```python
from build123d import *

# Parameters (mm, degrees)
SKETCH1_W           = 20
SKETCH1_H           = 13
BOSS_EXTRUDE1_DEPTH = 3
SKETCH2_W           = 20
SKETCH2_H           = 3
BOSS_EXTRUDE2_DEPTH = 13
BOSS_EXTRUDE3_DEPTH = 3
CUT_EXTRUDE1_DEPTH  = 40.66221139


with BuildPart() as part:
    # Sketch1 → Boss-Extrude1 (new body)
    with BuildSketch(Plane.XY):
        with Locations((24.886831503, -27.055)):
            Rectangle(SKETCH1_W, SKETCH1_H)
    extrude(amount=BOSS_EXTRUDE1_DEPTH)

    # Sketch2 → Boss-Extrude2 (add)
    with BuildSketch(Plane.XY.offset(3)):
        with Locations((24.886831503, -22.055)):
            Rectangle(SKETCH2_W, SKETCH2_H)
    extrude(amount=BOSS_EXTRUDE2_DEPTH)

    # Sketch3 → Boss-Extrude3 (add)
    with BuildSketch(Plane(origin=(34.886831503, 0, 0), x_dir=(0, 0, -1), z_dir=(1, 0, 0))):
        Polygon((-7.239132511, -23.555), (-3, -27.79413251), (-3, -23.554999999), align=None)
    boss_extrude3 = extrude(amount=-BOSS_EXTRUDE3_DEPTH)

    # Sketch4 → Cut-Extrude1 (cut, through all)
    with BuildSketch(Plane.XZ.offset(23.555)):
        with BuildLine():
            Line((28.386831503, 4.812110779), (28.386831503, 13.441160462))
            ThreePointArc((28.386831503, 13.441160462), (29.886831503, 14.941160462), (31.386831503, 13.441160462))
            Line((31.386831503, 13.441160462), (31.386831503, 4.812110779))
            ThreePointArc((31.386831503, 4.812110779), (29.886831503, 3.312110779), (28.386831503, 4.812110779))
        make_face()
    cut_extrude1 = extrude(amount=-CUT_EXTRUDE1_DEPTH, mode=Mode.SUBTRACT)

    # Mirror1: Boss-Extrude3, Cut-Extrude1 across plane
    add(boss_extrude3.mirror(Plane.ZY.offset(-24.886831503)))
    add(cut_extrude1.mirror(Plane.ZY.offset(-24.886831503)), mode=Mode.SUBTRACT)


solid = part.part
```
Check sheet for the modelled part. Datum: model origin and axes. Units: mm. A direction names the side the tool comes from. Round coordinates to 2 decimals unless told otherwise and drop trailing zeros. Order: outer loops, then holes, each group sorted by start corner. A loop starts at its lowest first (then second) coordinate and runs counter-clockwise, first axis right, second up.
1) Section check A-A (y = -23.25). Record the boundary of the cut face in (x, z).
2) Section check C-C (x = 20.5). Record the boundary of the cut face in (y, z) (3 decimals).
3) Go/stop test with a flat-tipped pin: pin 1 Ø4 at (x, z) = (29.5, 9.5) entering from -Y (3 decimals). Record where the tip stops, or that it passes through.
4) Tool access check on faces 4 (the flat face through (28.387, -22, 9)), 5 (the flat face through (25, -23.555, 9)), 6 (the flat face through (25, -20.555, 8)). Record the directions out of +Z, -Z, +X, -X, +Y, -Y that give a thin tool (end or side, any length) a straight path to the whole face; none if there is none.
5) Scan lines: line 1 (X direction, y = -23, z = 4.75); line 2 (X direction, y = -24.5, z = 4); line 3 (Z direction, x = 22.5, y = -29.5). Record each from-to range of solid material in increasing order.
6) Section check B-B (z = 12). Record the boundary of the cut face in (x, y) (3 decimals).
7) Section check D-D (x = 33.25). Record the boundary of the cut face in (y, z) (3 decimals).
8) Mould release check, pull along X, two halves, no side actions. Record for faces 1 (the cylindrical face through (29.85, -22.08, 14.94)), 2 (the flat face through (16.366, -25.645, 5.149)), 3 (the flat face through (34.887, -24, 5)): +X half, -X half, draft (parallel to the pull), parting line (faces both ways), or undercut.
Result:
1. outline: (14.89, 0) - (34.89, 0) - (34.89, 16) - (14.89, 16) - close; hole (18.39, 4.81) arc R1.5 ccw to (21.39, 4.81) - (21.39, 13.44) arc R1.5 ccw to (18.39, 13.44) - close; hole (28.39, 4.81) arc R1.5 ccw to (31.39, 4.81) - (31.39, 13.44) arc R1.5 ccw to (28.39, 13.44) - close
2. outline: (-33.555, 0) - (-20.555, 0) - (-20.555, 3.443) - (-23.555, 3.443) - (-23.555, 3) - (-33.555, 3) - close; (-23.555, 14.81) - (-20.555, 14.81) - (-20.555, 16) - (-23.555, 16) - close
3. pin 1: stops at y = -23.555
4. face 4: +Y, -Y
4. face 5: +Z, -Y
4. face 6: +Z, -Z, +X, -X, +Y
5. line 1: x = 14.89 to 18.39, 21.39 to 28.39, 31.39 to 34.89
5. line 2: x = 14.89 to 17.89, 31.89 to 34.89
5. line 3: z = 0 to 3
6. outline: (14.887, -23.555) - (18.387, -23.555) - (18.387, -20.555) - (14.887, -20.555) - close; (21.387, -23.555) - (28.387, -23.555) - (28.387, -20.555) - (21.387, -20.555) - close; (31.387, -23.555) - (34.887, -23.555) - (34.887, -20.555) - (31.387, -20.555) - close
7. outline: (-33.555, 0) - (-20.555, 0) - (-20.555, 16) - (-23.555, 16) - (-23.555, 7.239) - (-27.794, 3) - (-33.555, 3) - close
8. face 1: undercut
8. face 2: draft
8. face 3: +X half
